```python
from build123d import *

# Parameters (mm, degrees)
SKETCH_1_R               = 1.265
EXTRUDE_1_DEPTH          = 10
SKETCH_2_R               = 2.75
SKETCH_2_R_2             = 1.225
EXTRUDE_2_DEPTH          = 1.2
SKETCH_3_R               = 10.210079725
SKETCH_3_R_2             = 7.3
CUT_EXTRUDE_2_DEPTH      = 16.316956182
FILLET_1_R               = 0.5
PATTERN_CIRCULAR_2_DEPTH = 10


# Read off the part's stored shape, not the designer's step: Круговой массив2
with BuildPart() as part:
    # Эскиз1 → Бобышка-Вытянуть1 (new body)
    with BuildSketch(Plane.XY):
        with BuildLine():
            ThreePointArc((-3.148803906, 3.471068454), (-4.227852242, 4.566214035), (-5.743712894, 4.822837566))
            ThreePointArc((-5.743712894, 4.822837566), (-5.841480421, 4.703945843), (-5.936787387, 4.583072716))
            ThreePointArc((-5.936787387, 4.583072716), (-5.362797198, 3.156810321), (-4.062728379, 2.336133637))
            ThreePointArc((-4.062728379, 2.336133637), (-4.379801209, 1.667520202), (-4.587678719, 0.95733287))
            ThreePointArc((-4.587678719, 0.95733287), (-6.104357582, 1.209075557), (-7.481554138, 0.525687819))
            ThreePointArc((-7.481554138, 0.525687819), (-7.490766927, 0.372036085), (-7.496824441, 0.218227641))
            ThreePointArc((-7.496824441, 0.218227641), (-6.194120622, -0.598259906), (-4.659961201, -0.498040012))
            ThreePointArc((-4.659961201, -0.498040012), (-4.523477392, -1.225330377), (-4.274216191, -1.922071332))
            ThreePointArc((-4.274216191, -1.922071332), (-5.649205805, -2.609888688), (-6.361695989, -3.972256807))
            ThreePointArc((-6.361695989, -3.972256807), (-6.278835069, -4.101978813), (-6.193329365, -4.229972975))
            ThreePointArc((-6.193329365, -4.229972975), (-4.659500498, -4.124815183), (-3.477247231, -3.141979304))
            ThreePointArc((-3.477247231, -3.141979304), (-2.939338959, -3.650146399), (-2.328148353, -4.067309614))
            ThreePointArc((-2.328148353, -4.067309614), (-3.03624942, -5.431964161), (-2.811886199, -6.952934345))
            ThreePointArc((-2.811886199, -6.952934345), (-2.668601624, -7.009177225), (-2.524192976, -7.062467686))
            ThreePointArc((-2.524192976, -7.062467686), (-1.345109555, -6.075831258), (-0.966343005, -4.585789294))
            ThreePointArc((-0.966343005, -4.585789294), (-0.232472948, -4.68073056), (0.507193024, -4.658973866))
            ThreePointArc((0.507193024, -4.658973866), (0.736451045, -6.179213951), (1.811968547, -7.277827285))
            ThreePointArc((1.811968547, -7.277827285), (1.960946938, -7.239108171), (2.109099336, -7.197339786))
            ThreePointArc((2.109099336, -7.197339786), (2.483067519, -5.706086302), (1.913671403, -4.277983638))
            ThreePointArc((1.913671403, -4.277983638), (2.563189827, -3.92343474), (3.148803906, -3.471068454))
            ThreePointArc((3.148803906, -3.471068454), (4.227852242, -4.566214035), (5.743712894, -4.822837566))
            ThreePointArc((5.743712894, -4.822837566), (5.841480421, -4.703945843), (5.936787387, -4.583072716))
            ThreePointArc((5.936787387, -4.583072716), (5.362797198, -3.156810321), (4.062728379, -2.336133637))
            ThreePointArc((4.062728379, -2.336133637), (4.379801209, -1.667520202), (4.587678719, -0.95733287))
            ThreePointArc((4.587678719, -0.95733287), (6.104357582, -1.209075557), (7.481554138, -0.525687819))
            ThreePointArc((7.481554138, -0.525687819), (7.490766927, -0.372036085), (7.496824441, -0.218227641))
            ThreePointArc((7.496824441, -0.218227641), (6.194120622, 0.598259906), (4.659961201, 0.498040012))
            ThreePointArc((4.659961201, 0.498040012), (4.523477392, 1.225330377), (4.274216191, 1.922071332))
            ThreePointArc((4.274216191, 1.922071332), (5.649205805, 2.609888688), (6.361695989, 3.972256807))
            ThreePointArc((6.361695989, 3.972256807), (6.278835069, 4.101978813), (6.193329365, 4.229972975))
            ThreePointArc((6.193329365, 4.229972975), (4.659500498, 4.124815183), (3.477247231, 3.141979304))
            ThreePointArc((3.477247231, 3.141979304), (2.939338959, 3.650146399), (2.328148353, 4.067309614))
            ThreePointArc((2.328148353, 4.067309614), (3.03624942, 5.431964161), (2.811886199, 6.952934345))
            ThreePointArc((2.811886199, 6.952934345), (2.668601624, 7.009177225), (2.524192976, 7.062467686))
            ThreePointArc((2.524192976, 7.062467686), (1.345109555, 6.075831258), (0.966343005, 4.585789294))
            ThreePointArc((0.966343005, 4.585789294), (0.232472948, 4.68073056), (-0.507193024, 4.658973866))
            ThreePointArc((-0.507193024, 4.658973866), (-0.736451045, 6.179213951), (-1.811968547, 7.277827285))
            ThreePointArc((-1.811968547, 7.277827285), (-1.960946938, 7.239108171), (-2.109099336, 7.197339786))
            ThreePointArc((-2.109099336, 7.197339786), (-2.483067519, 5.706086302), (-1.913671403, 4.277983638))
            ThreePointArc((-1.913671403, 4.277983638), (-2.563189827, 3.92343474), (-3.148803906, 3.471068454))
        make_face()
        Circle(SKETCH_1_R, mode=Mode.SUBTRACT)
    extrude(amount=EXTRUDE_1_DEPTH)

    # Эскиз2 → Бобышка-Вытянуть2 (add)
    with BuildSketch(Plane.XY.offset(10)):
        Circle(SKETCH_2_R)
        Circle(SKETCH_2_R_2, mode=Mode.SUBTRACT)
    extrude(amount=EXTRUDE_2_DEPTH)

    # Эскиз3 → Вырез-Вытянуть2 (cut, through all)
    with BuildSketch(Plane(origin=(0, 0, 0), x_dir=(-1, 0, 0), z_dir=(0, 0, -1))):
        Circle(SKETCH_3_R)
        Circle(SKETCH_3_R_2, mode=Mode.SUBTRACT)
    extrude(amount=-CUT_EXTRUDE_2_DEPTH, mode=Mode.SUBTRACT)

    # Скругление1
    fillet_1_edges = [part.edges().sort_by_distance(p)[0] for p in [
        (-2.246892365, 6.945608303, 5),
        (-1.565958675, 7.13006125, 5),
    ]]
    fillet(fillet_1_edges, radius=FILLET_1_R)

    # Круговой массив2 outline → Круговой массив2 (cut)
    with BuildSketch(Plane.XY):
        with BuildLine():
            ThreePointArc((-5.838293306, 4.042408612), (-5.850561559, 4.278183981), (-5.753278974, 4.493304024))
            ThreePointArc((-5.753278974, 4.493304024), (-5.827604273, 4.396479095), (-5.900300237, 4.298424958))
            ThreePointArc((-5.900300237, 4.298424958), (-5.872671085, 4.169599529), (-5.838293306, 4.042408612))
        make_face()
        with BuildLine():
            ThreePointArc((-5.457832031, 4.847893307), (-5.538127486, 4.755958783), (-5.61687454, 4.662694543))
            ThreePointArc((-5.61687454, 4.662694543), (-5.427449488, 4.803615386), (-5.19448163, 4.841910441))
            ThreePointArc((-5.19448163, 4.841910441), (-5.326077976, 4.84837285), (-5.457832031, 4.847893307))
        make_face()
        with BuildLine():
            ThreePointArc((-7.099346669, -0.161285439), (-7.247857179, 0.022249743), (-7.295598302, 0.253466783))
            ThreePointArc((-7.295598302, 0.253466783), (-7.298816468, 0.131446456), (-7.299993962, 0.009389377))
            ThreePointArc((-7.299993962, 0.009389377), (-7.201919821, -0.078592576), (-7.099346669, -0.161285439))
        make_face()
        with BuildLine():
            ThreePointArc((-7.264999056, 0.713994895), (-7.275921686, 0.592421818), (-7.284810046, 0.470683106))
            ThreePointArc((-7.284810046, 0.470683106), (-7.214393154, 0.696031715), (-7.048427465, 0.863948137))
            ThreePointArc((-7.048427465, 0.863948137), (-7.158689654, 0.791825944), (-7.264999056, 0.713994895))
        make_face()
        with BuildLine():
            ThreePointArc((-5.648690902, -4.303373934), (-5.876717701, -4.24218314), (-6.051247048, -4.083186154))
            ThreePointArc((-6.051247048, -4.083186154), (-5.982128849, -4.183794263), (-5.911338111, -4.283232627))
            ThreePointArc((-5.911338111, -4.283232627), (-5.78027997, -4.296764989), (-5.648690902, -4.303373934))
        make_face()
        with BuildLine():
            ThreePointArc((-6.29718337, -3.692625299), (-6.234561102, -3.797400146), (-6.170195716, -3.90111328))
            ThreePointArc((-6.170195716, -3.90111328), (-6.245683843, -3.677412414), (-6.210113576, -3.444012991))
            ThreePointArc((-6.210113576, -3.444012991), (-6.2569252, -3.567171559), (-6.29718337, -3.692625299))
        make_face()
        with BuildLine():
            ThreePointArc((-2.040427202, -6.801719852), (-2.260871804, -6.88624625), (-2.495525095, -6.860200762))
            ThreePointArc((-2.495525095, -6.860200762), (-2.380471335, -6.900967774), (-2.264752021, -6.939805349))
            ThreePointArc((-2.264752021, -6.939805349), (-2.150769635, -6.873719217), (-2.040427202, -6.801719852))
        make_face()
        with BuildLine():
            ThreePointArc((-2.92405767, -6.688788137), (-2.811810081, -6.736744322), (-2.69877634, -6.782816986))
            ThreePointArc((-2.69877634, -6.782816986), (-2.891335587, -6.646209992), (-2.999747375, -6.436478214))
            ThreePointArc((-2.999747375, -6.436478214), (-2.965227985, -6.563630771), (-2.92405767, -6.688788137))
        make_face()
        with BuildLine():
            ThreePointArc((2.347210337, -6.702039969), (2.218550278, -6.899997348), (2.013402624, -7.016851849))
            ThreePointArc((2.013402624, -7.016851849), (2.130445319, -6.982206151), (2.246892365, -6.945608303))
            ThreePointArc((2.246892365, -6.945608303), (2.300261598, -6.825146334), (2.347210337, -6.702039969))
        make_face()
        with BuildLine():
            ThreePointArc((1.565958675, -7.13006125), (1.684956821, -7.102881142), (1.80348387, -7.073715143))
            ThreePointArc((1.80348387, -7.073715143), (1.56740459, -7.076381249), (1.356420365, -6.970427527))
            ThreePointArc((1.356420365, -6.970427527), (1.459085537, -7.053006118), (1.565958675, -7.13006125))
        make_face()
        with BuildLine():
            ThreePointArc((5.838293306, -4.042408612), (5.850561559, -4.278183981), (5.753278974, -4.493304024))
            ThreePointArc((5.753278974, -4.493304024), (5.827604273, -4.396479095), (5.900300237, -4.298424958))
            ThreePointArc((5.900300237, -4.298424958), (5.872671085, -4.169599529), (5.838293306, -4.042408612))
        make_face()
        with BuildLine():
            ThreePointArc((5.457832031, -4.847893307), (5.538127486, -4.755958783), (5.61687454, -4.662694543))
            ThreePointArc((5.61687454, -4.662694543), (5.427449488, -4.803615386), (5.19448163, -4.841910441))
            ThreePointArc((5.19448163, -4.841910441), (5.326077976, -4.84837285), (5.457832031, -4.847893307))
        make_face()
        with BuildLine():
            ThreePointArc((7.099346669, 0.161285439), (7.247857179, -0.022249743), (7.295598302, -0.253466783))
            ThreePointArc((7.295598302, -0.253466783), (7.298816468, -0.131446456), (7.299993962, -0.009389377))
            ThreePointArc((7.299993962, -0.009389377), (7.201919821, 0.078592576), (7.099346669, 0.161285439))
        make_face()
        with BuildLine():
            ThreePointArc((7.264999056, -0.713994895), (7.275921686, -0.592421818), (7.284810046, -0.470683106))
            ThreePointArc((7.284810046, -0.470683106), (7.214393154, -0.696031715), (7.048427465, -0.863948137))
            ThreePointArc((7.048427465, -0.863948137), (7.158689654, -0.791825944), (7.264999056, -0.713994895))
        make_face()
        with BuildLine():
            ThreePointArc((5.648690902, 4.303373934), (5.876717701, 4.24218314), (6.051247048, 4.083186154))
            ThreePointArc((6.051247048, 4.083186154), (5.982128849, 4.183794263), (5.911338111, 4.283232627))
            ThreePointArc((5.911338111, 4.283232627), (5.78027997, 4.296764989), (5.648690902, 4.303373934))
        make_face()
        with BuildLine():
            ThreePointArc((6.29718337, 3.692625299), (6.234561102, 3.797400146), (6.170195716, 3.90111328))
            ThreePointArc((6.170195716, 3.90111328), (6.245683843, 3.677412414), (6.210113576, 3.444012991))
            ThreePointArc((6.210113576, 3.444012991), (6.2569252, 3.567171559), (6.29718337, 3.692625299))
        make_face()
        with BuildLine():
            ThreePointArc((2.040427202, 6.801719852), (2.260871804, 6.88624625), (2.495525095, 6.860200762))
            ThreePointArc((2.495525095, 6.860200762), (2.380471335, 6.900967774), (2.264752021, 6.939805349))
            ThreePointArc((2.264752021, 6.939805349), (2.150769635, 6.873719217), (2.040427202, 6.801719852))
        make_face()
        with BuildLine():
            ThreePointArc((2.92405767, 6.688788137), (2.811810081, 6.736744322), (2.69877634, 6.782816986))
            ThreePointArc((2.69877634, 6.782816986), (2.891335587, 6.646209992), (2.999747375, 6.436478214))
            ThreePointArc((2.999747375, 6.436478214), (2.965227985, 6.563630771), (2.92405767, 6.688788137))
        make_face()
    extrude(amount=PATTERN_CIRCULAR_2_DEPTH, mode=Mode.SUBTRACT)


solid = part.part
```
Verification items for the finished model (mm, model axes). Coordinates: 2 decimals unless noted, no trailing zeros. Write each loop counter-clockwise with the first axis right and the second up, starting at its lowest first coordinate (ties: lowest second). Pieces come first, ordered by that corner, then holes. Notation, with made-up numbers: (62.5, 84.5) - (89.5, 84.5) arc R18 ccw to (89.5, 111.5) - close; hole circle Ø1 at (68.25, 52). An arc over 180 degrees is marked (long way). One line per question, with ' | ' between items. Start each with the question number.
1. Section check C-C (y = 5.25). Enter the section's corners in (x, z), plus the area to 3 significant figures.
2. Draft check along X on faces 1 (the cylindrical face through (4.376, -1.677, 4.93)), 2 (the flat face through (1, -1, 11.2)). Enter one of: released by +X, released by -X, zero draft, split by the parting line, or undercut.
3. Gauge pin test, flat ends, axial feed: P1, Ø3, axis at x = 5.5, z = 3, coming from the -Y side; P2, Ø1, axis at x = -4, z = 5.5, coming from the +Y side; P3, Ø1.5, axis at x = 0, y = 0, coming from the +Z side. Record the tip position at first contact, or that the pin passes through.
4. Material ranges on line 1 along Y through (x, z) = (0, 7.75) (1 decimal); line 2 along Z through (x, y) = (5.25, 3.75); line 3 along Y through (x, z) = (-5.5, 4.25), recorded low to high.
5. Section check B-B (y = -6). Enter the section's corners in (x, z).
Computed values:
1) outline: (-2.41, 0) - (-0.48, 0) - (-0.48, 10) - (-2.41, 10) - close; (1.01, 0) - (3, 0) - (3, 10) - (1.01, 10) - close | area: 39.1 mm²
2) face 1: undercut | face 2: zero draft
3) P1: y = -4.84 | P2: y = 4.69 | P3: through
4) line 1: -4.7 to -1.3, 1.3 to 4.7 | line 2: 0 to 10 | line 3: -4.3 to -2.47, -0.67 to 1.23, 3.34 to 4.77
5) outline: (-3.07, 0) - (-1.3, 0) - (-1.3, 10) - (-3.07, 10) - close; (0.66, 0) - (2.49, 0) - (2.49, 10) - (0.66, 10) - close
